Answer from the drawing. Dimensions are ordinates in mm from the lowest x, y and z of the part. A direction names the side the tool comes from. Round coordinates to 2 decimals unless told otherwise and drop trailing zeros. Write each loop counter-clockwise with the first axis right and the second up, starting at its lowest first coordinate (ties: lowest second). Pieces come first, ordered by that corner, then holes. Notation, with made-up numbers: (76.25, 27.25) - (110.25, 27.25) arc R6 ccw to (110.25, 37.25) - close; hole circle Ø10 at (21, 67). An arc over 180 degrees is marked (long way). Use a Markdown table: item, result. Add a question column.
1) Each of these flat-tipped pins is pushed along its axis until it touches: P1, Ø3.5, axis at y = 3, z = 62, coming from the +X side; P2, Ø3, axis at x = 271.5, y = 7.5, coming from the -Z side; P3, Ø1, axis at y = 6, z = 50.5, coming from the +X side. Where does it stop, or does it pass through?
2) A cutting plane is placed at A-A (y = 7). State how many separate pieces and enclosed holes the cut face has, then the cut area to 3 significant figures.
3) A cutting plane is placed at C-C (z = 38.1). Give the vertices of the cut face in (x, y) (1 decimal), then the cut area to 3 significant figures.
4) A cutting plane is placed at D-D (x = 182). Give the vertices of the cut face in (y, z) (1 decimal), then the cut area to 3 significant figures.
5) Find the intervals of material crossed by probe 1 along Z at (x, y) = (153, 6); probe 2 along X at (y, z) = (5.5, 15) (1 decimal); probe 3 along X at (y, z) = (6.5, 52) (1 decimal), in increasing order. Write a range as from..to.
6) A tool of negligible diameter and unlimited length cuts with its end or side. For the marked faces 1 and 2, from which of +Z, -Z, +X, -X, +Y, -Y can it reach the whole face along a straight path? Write none if from no direction.
7) Determine the mould class of the marked faces 3 and 4 for opening direction X: +X half, -X half, draft (parallel to the pull), parting line (faces both ways), or undercut.
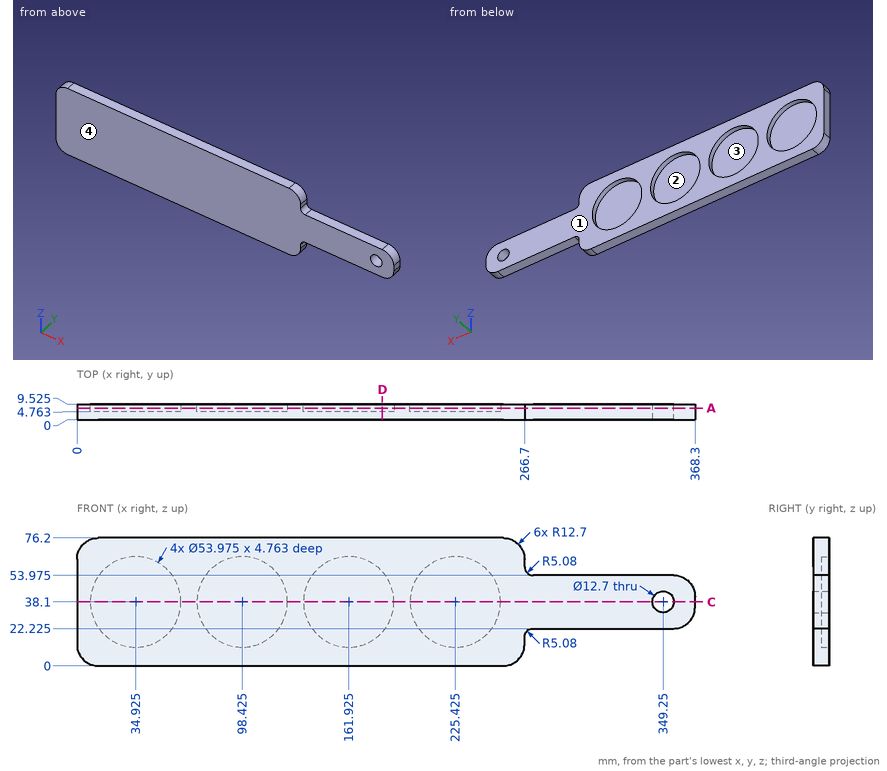
Entries:
| question | item | result |
|---|---|---|
| 1 | P1 | stops at x = 266.7 |
| 1 | P2 | stops at z = 21.9 |
| 1 | P3 | stops at x = 364.83 |
| 2 | separate pieces | 1 |
| 2 | enclosed holes | 5 |
| 2 | area | 14,100 mm² |
| 3 | outline | (0, 0) - (342.9, 0) - (342.9, 9.5) - (252.4, 9.5) - (252.4, 4.8) - (198.4, 4.8) - (198.4, 9.5) - (188.9, 9.5) - (188.9, 4.8) - (134.9, 4.8) - (134.9, 9.5) - (125.4, 9.5) - (125.4, 4.8) - (71.4, 4.8) - (71.4, 9.5) - (61.9, 9.5) - (61.9, 4.8) - (7.9, 4.8) - (7.9, 9.5) - (0, 9.5) - close; (355.6, 0) - (368.3, 0) - (368.3, 9.5) - (355.6, 9.5) - close |
| 3 | area | 2,360 mm² |
| 4 | outline | (0, 0) - (9.5, 0) - (9.5, 20.1) - (4.8, 20.1) - (4.8, 56.1) - (9.5, 56.1) - (9.5, 76.2) - (0, 76.2) - close |
| 4 | area | 554 mm² |
| 5 | probe 1 | z = 0..12.63, 63.57..76.2 |
| 5 | probe 2 | x = 0..21, 48.9..84.5, 112.4..148, 175.9..211.5, 239.4..266.7 |
| 5 | probe 3 | x = 0..11.8, 58.1..75.3, 121.6..138.8, 185.1..202.3, 248.6..362.4 |
| 6 | face 1 | +Z, -Z, +X, -X, +Y |
| 6 | face 2 | +Y |
| 7 | face 3 | undercut |
| 7 | face 4 | draft |
